The drawing under review shows one solid part. Ordinate dimensions are in mm from its lowest x, y, z. Round coordinates to 2 decimals unless told otherwise and drop trailing zeros. Order: outer loops, then holes, each group sorted by start corner. A loop starts at its lowest first (then second) coordinate and runs counter-clockwise, first axis right, second up. Notation, with made-up numbers: M 8,8.5 L 48,8.5 A10 cw 48,23.5 Z; hole C 76.25,76.25 d2. An arc over 180 degrees is marked long. Answer in a Markdown table with one row per item. Add a question column.
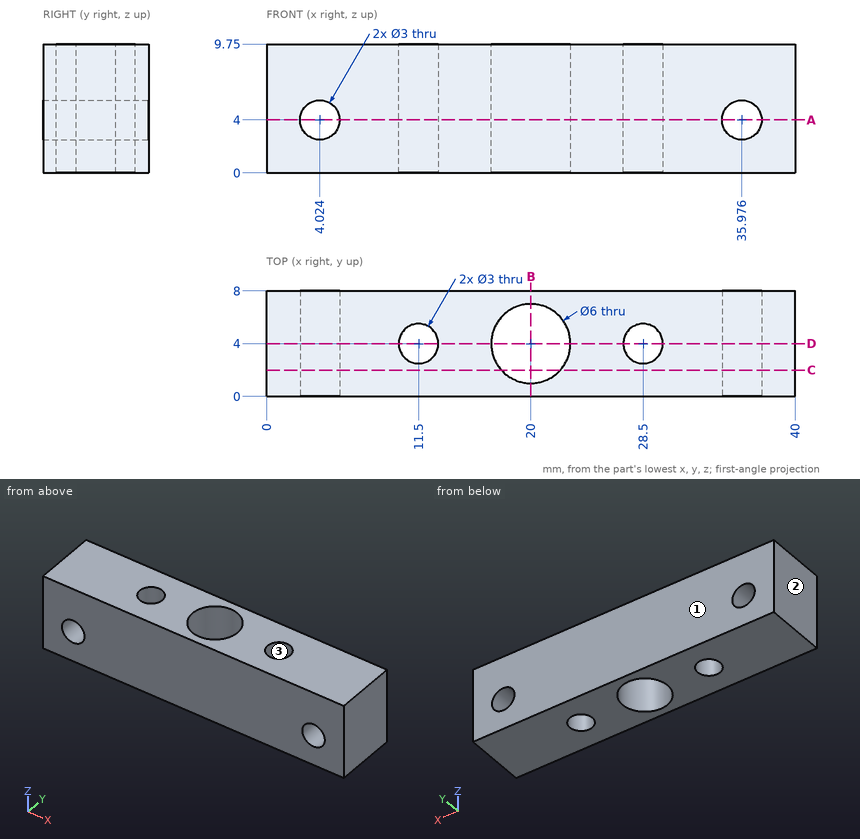
1. Consider section B-B on x = 20. Write out the cut boundary in (y, z), plus the area to 3 significant figures.
2. Clearance check with flat-ended pins moving along their axes: pin 1 Ø3.5 at (x, z) = (4.02, 4) entering from +Y; pin 2 Ø3.5 at (x, y) = (20, 4) entering from -Z. State where each tip first meets the part, or that it passes through.
3. The part is to be moulded in two halves that separate along Y. For the marked faces 1, 2 and 3, say which applies: pulls with the +Y half, pulls with the -Y half, needs draft (parallel to the pull), parting line crosses it, or undercut.
4. Consider section A-A on z = 4. Write out the cut boundary in (x, y), plus the area to 3 significant figures.
5. To check wall thickness, follow probe 1 along Y at (x, z) = (28.5, 2.5); probe 2 along X at (y, z) = (2, 4); probe 3 along Z at (x, y) = (4, 0.5). State the ranges of each line that lie inside material, in increasing order. Write a range as [from, to].
6. Consider section C-C on y = 2. Write out the cut boundary in (x, z), plus the area to 3 significant figures.
7. Consider section D-D on y = 4. Write out the cut boundary in (x, z), plus the area to 3 significant figures.
Solved:
| question | item | result |
|---|---|---|
| 1 | outline | M 0,0 L 1,0 L 1,9.75 L 0,9.75 Z; M 7,0 L 8,0 L 8,9.75 L 7,9.75 Z |
| 1 | area | 19.5 mm^2 |
| 2 | pin 1 | stops at y = 8 |
| 2 | pin 2 | passes through |
| 3 | face 1 | pulls with the +Y half |
| 3 | face 2 | needs draft |
| 3 | face 3 | undercut |
| 4 | outline | M 0,0 L 2.52,0 L 2.52,8 L 0,8 Z; M 5.52,0 L 34.48,0 L 34.48,8 L 5.52,8 Z; M 37.48,0 L 40,0 L 40,8 L 37.48,8 Z; hole C 11.5,4 d3; hole C 20,4 d6; hole C 28.5,4 d3 |
| 4 | area | 230 mm^2 |
| 5 | probe 1 | y = [0, 2.5], [5.5, 8] |
| 5 | probe 2 | x = [0, 2.52], [5.52, 17.76], [22.24, 34.48], [37.48, 40] |
| 5 | probe 3 | z = [0, 2.5], [5.5, 9.75] |
| 6 | outline | M 0,0 L 17.76,0 L 17.76,9.75 L 0,9.75 Z; M 22.24,0 L 40,0 L 40,9.75 L 22.24,9.75 Z; hole C 4.02,4 d3; hole C 35.98,4 d3 |
| 6 | area | 332 mm^2 |
| 7 | outline | M 0,0 L 10,0 L 10,9.75 L 0,9.75 Z; M 13,0 L 17,0 L 17,9.75 L 13,9.75 Z; M 23,0 L 27,0 L 27,9.75 L 23,9.75 Z; M 30,0 L 40,0 L 40,9.75 L 30,9.75 Z; hole C 4.02,4 d3; hole C 35.98,4 d3 |
| 7 | area | 259 mm^2 |
